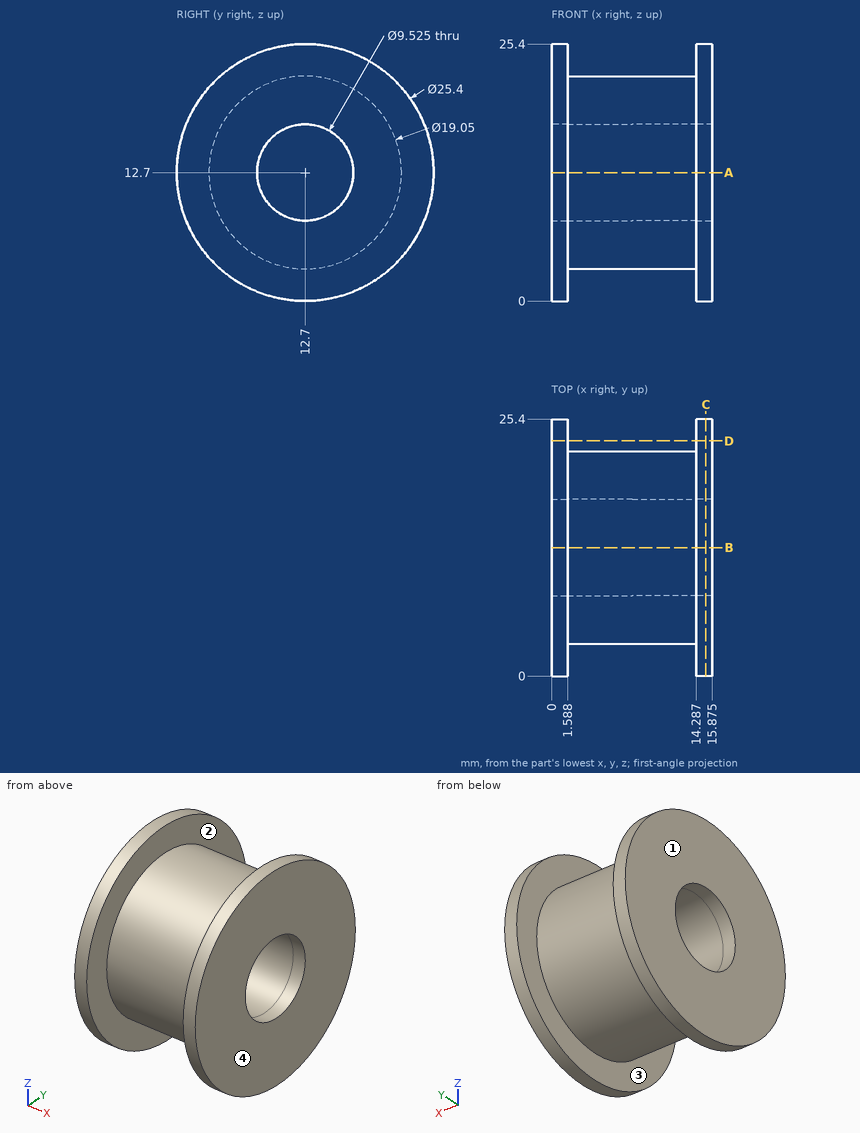
The figure shows three views and two pictorial views of one solid part (mm, origin at its lowest corner). Answer the questions. Round coordinates to 2 decimals unless told otherwise and drop trailing zeros. Loops run counter-clockwise (first coordinate to the right, second up) from the corner with the lowest first, then second, coordinate; pieces in that order, holes last. Notation, with made-up numbers: (35, 61.25) - (85, 61.25) arc R27 cw to (85, 84.25) - close; hole circle Ø2 at (-22.5, 5.5). An arc over 180 degrees is marked (long way). Use one line per item in the form item = value. Start each with the question number.
(1) Consider line 1 (X direction, y = 4.5, z = 7.75) (1 decimal); line 2 (Y direction, x = 15, z = 12.7); line 3 (Z direction, x = 11.5, y = 12.7) (1 decimal). Determine where each line is inside the solid, lowest interval first.
(2) Find section D-D on y = 23.25. Determine the outline of the cut face in (x, z) (1 decimal).
(3) Determine the mould class of the marked faces 1, 2, 3 and 4 for opening direction X: +X half, -X half, draft (parallel to the pull), parting line (faces both ways), or undercut.
(4) Find section A-A on z = 12.7. Determine the outline of the cut face in (x, y) (1 decimal), and give its area (3 significant figures).
(5) Find section C-C on x = 15.25. Determine the outline of the cut face in (y, z) (1 decimal).
(6) Flat-ended cylindrical pins translate along their axes: P1, Ø8, axis at x = 12, z = 8, coming from the +Y side; P2, Ø3, axis at x = 7, z = 3.5, coming from the +Y side (1 decimal); P3, Ø4, axis at x = 12, y = 15.5, coming from the -Z side. Find the tip coordinate at first contact, or state that the pin passes through.
Answer list:
q1.line_1 = 0 to 1.6, 14.3 to 15.9
q1.line_2 = 0 to 7.94, 17.46 to 25.4
q1.line_3 = 3.2 to 7.9, 17.5 to 22.2
q2.outline = (0, 5.6) - (1.6, 5.6) - (1.6, 19.8) - (0, 19.8) - close; (14.3, 5.6) - (15.9, 5.6) - (15.9, 19.8) - (14.3, 19.8) - close
q3.face_1 = -X half
q3.face_2 = undercut
q3.face_3 = undercut
q3.face_4 = +X half
q4.outline = (0, 0) - (1.6, 0) - (1.6, 3.2) - (14.3, 3.2) - (14.3, 0) - (15.9, 0) - (15.9, 7.9) - (0, 7.9) - close; (0, 17.5) - (15.9, 17.5) - (15.9, 25.4) - (14.3, 25.4) - (14.3, 22.2) - (1.6, 22.2) - (1.6, 25.4) - (0, 25.4) - close
q4.area = 171 mm^2
q5.outline = circle Ø25.4 at (12.7, 12.7); hole circle Ø9.5 at (12.7, 12.7)
q6.P1 = 25.32
q6.P2 = 18.3
q6.P3 = 3.21
